The listing builds one solid part. Answer for the finished solid, in the listing's coordinates (mm). A direction names the side the tool comes from. Coordinates: 2 decimals unless noted, no trailing zeros. Write each loop counter-clockwise with the first axis right and the second up, starting at its lowest first coordinate (ties: lowest second). Pieces come first, ordered by that corner, then holes.
from build123d import *
from build123d.topology import SkipClean

# Parameters (mm, degrees)
SKETCH_1_W          = 60
SKETCH_1_H          = 60
EXTRUDE_1_DEPTH     = 5
EXTRUDE_START       = 5
SKETCH_2_R          = 17.67766953
EXTRUDE_3_DEPTH     = 10
SKETCH_6_W          = 30
SKETCH_6_H          = 30
CUT_EXTRUDE_2_DEPTH = 5
CHAMFER_1_SIZE      = 5
SKETCH_7_R          = 6.25
EXTRUDE_4_DEPTH     = 7
CUT_EXTRUDE_START   = 5
CUT_EXTRUDE_3_DEPTH = 5
CUT_EXTRUDE_4_DEPTH = 7
SKETCH_18_R         = 2.5
CUT_EXTRUDE_5_DEPTH = 12
SKETCH_21_R         = 2.5
CUT_EXTRUDE_6_DEPTH = 10
FILLET_1_R          = 1
FILLET_2_R          = 3


with BuildPart() as part:
    # 草图1 → 凸台-拉伸1 (new body)
    with BuildSketch(Plane(origin=(0, 0, 0), x_dir=(1, 0, 0), z_dir=(0, 1, 0))):
        Rectangle(SKETCH_1_W, SKETCH_1_H)
    extrude(amount=EXTRUDE_1_DEPTH)

    # 草图2 → 凸台-拉伸3 (add)
    with BuildSketch(Plane(origin=(0, 0, 0), x_dir=(1, 0, 0), z_dir=(0, 1, 0)).offset(EXTRUDE_START)):
        with Locations(Location((0, 0, 0), (0, 0, 90))):
            Circle(SKETCH_2_R)
    extrude(amount=EXTRUDE_3_DEPTH)

    # 扫描1: sweep along a curve in space
    with BuildLine() as sweep_1_path:
        ThreePointArc((0, 5, -17.67766953), (12.5, 5, -12.5), (17.67766953, 5, 0))
        ThreePointArc((17.67766953, 5, 0), (12.5, 5, 12.5), (0, 5, 17.67766953))
        ThreePointArc((0, 5, 17.67766953), (-12.5, 5, 12.5), (-17.67766953, 5, 0))
        ThreePointArc((-17.67766953, 5, 0), (-12.5, 5, -12.5), (0, 5, -17.67766953))
    # 草图4 → 扫描1 (sweep)
    with BuildSketch(Plane.XY):
        Polygon((17.67766953, 15), (17.67766953, 5), (27.67766953, 5), align=None)
    sweep(path=sweep_1_path.line)

    # 草图6 → 切除-拉伸2 (cut)
    with BuildSketch(Plane(origin=(0, 0, 0), x_dir=(1, 0, 0), z_dir=(0, 1, 0))):
        Rectangle(SKETCH_6_W, SKETCH_6_H)
    extrude(amount=CUT_EXTRUDE_2_DEPTH, mode=Mode.SUBTRACT)

    # 倒角1
    chamfer_1_edges = [part.edges().sort_by_distance(p)[0] for p in [
        (0, 5, -15),
        (-15, 5, 0),
        (0, 5, 15),
        (15, 5, 0),
    ]]
    chamfer(chamfer_1_edges, length=CHAMFER_1_SIZE - 0.0001)  # a hair under: the kernel refuses the full size

    # 草图7 → 凸台-拉伸4 (add)
    with BuildSketch(Plane(origin=(0, 0, 0), x_dir=(1, 0, 0), z_dir=(0, 1, 0))):
        with Locations(Location((-23.75, 23.75, 0), (0, 0, 270))):
            Circle(SKETCH_7_R)
        with Locations(Location((23.75, 23.75, 0), (0, 0, 270))):
            Circle(SKETCH_7_R)
        with Locations(Location((-23.75, -23.75, 0), (0, 0, 270))):
            Circle(SKETCH_7_R)
        with Locations(Location((23.75, -23.75, 0), (0, 0, 270))):
            Circle(SKETCH_7_R)
    extrude(amount=-EXTRUDE_4_DEPTH)

    # 草图8 → 切除-拉伸3 (cut)
    with BuildSketch(Plane(origin=(0, 0, 0), x_dir=(1, 0, 0), z_dir=(0, 1, 0)).offset(CUT_EXTRUDE_START)):
        with BuildLine():
            Line((23.75, 30), (30, 30))
            Line((30, 30), (30, 23.75))
            ThreePointArc((30, 23.75), (28.169417382, 28.169417382), (23.75, 30))
        make_face()
        with BuildLine():
            Line((-30, 30), (-23.75, 30))
            ThreePointArc((-23.75, 30), (-28.169417382, 28.169417382), (-30, 23.75))
            Line((-30, 23.75), (-30, 30))
        make_face()
        with BuildLine():
            Line((-23.75, -30), (-30, -30))
            Line((-30, -30), (-30, -23.75))
            ThreePointArc((-30, -23.75), (-28.169417382, -28.169417382), (-23.75, -30))
        make_face()
        with BuildLine():
            Line((30, -23.75), (30, -30))
            Line((30, -30), (23.75, -30))
            ThreePointArc((23.75, -30), (28.169417382, -28.169417382), (30, -23.75))
        make_face()
    extrude(amount=-CUT_EXTRUDE_3_DEPTH, mode=Mode.SUBTRACT)

    # 草图9 → 旋转1 (revolve)
    with BuildSketch(Plane(origin=(0, 0, 23.75), x_dir=(-1, 0, 0), z_dir=(0, 0, -1)), mode=Mode.PRIVATE) as revolve_1_sk:
        Polygon((17.5, -7), (17.5, 0), (12.5, 0), align=None)
    revolve(revolve_1_sk.sketch.rotate(Axis((-23.75, 5, 23.75), (0, -1, 0)), 90), axis=Axis((-23.75, 5, 23.75), (0, -1, 0)))

    # 草图13 → 旋转2 (revolve)
    with BuildSketch(Plane(origin=(0, 0, 23.75), x_dir=(-1, 0, 0), z_dir=(0, 0, -1)), mode=Mode.PRIVATE) as revolve_2_sk:
        Polygon((-17.5, 0), (-17.5, -7), (-12.5, 0), align=None)
    revolve(revolve_2_sk.sketch.rotate(Axis((23.75, 5, 23.75), (0, -1, 0)), 270), axis=Axis((23.75, 5, 23.75), (0, -1, 0)))

    # 草图14 → 旋转3 (revolve)
    with BuildSketch(Plane(origin=(0, 0, -23.75), x_dir=(-1, 0, 0), z_dir=(0, 0, -1)), mode=Mode.PRIVATE) as revolve_3_sk:
        Polygon((-17.5, -7), (-12.5, 0), (-17.5, 0), align=None)
    revolve(revolve_3_sk.sketch.rotate(Axis((23.75, 5, -23.75), (0, -1, 0)), 270), axis=Axis((23.75, 5, -23.75), (0, -1, 0)))

    # 草图16 → 旋转4 (revolve)
    with BuildSketch(Plane(origin=(0, 0, -23.75), x_dir=(-1, 0, 0), z_dir=(0, 0, -1)), mode=Mode.PRIVATE) as revolve_4_sk:
        Polygon((17.5, 0), (17.5, -7), (12.5, 0), align=None)
    revolve(revolve_4_sk.sketch.rotate(Axis((-23.75, 5, -23.75), (0, -1, 0)), 90), axis=Axis((-23.75, 5, -23.75), (0, -1, 0)))

    # 草图17 → 切除-拉伸4 (cut)
    with SkipClean():  # the faces are left unmerged after this step: merging them gives an invalid solid
        with BuildSketch(Plane(origin=(0, 0, 0), x_dir=(1, 0, 0), z_dir=(0, 1, 0))):
            with BuildLine():
                Line((-30, -23.75), (-30, -14.395856533))
                ThreePointArc((-30, -14.395856533), (-31.704951288, -31.704951288), (-14.395856533, -30))
                Line((-14.395856533, -30), (-23.75, -30))
                ThreePointArc((-23.75, -30), (-28.169417382, -28.169417382), (-30, -23.75))
            make_face()
            with BuildLine():
                Line((30, -14.395856533), (30, -23.75))
                ThreePointArc((30, -23.75), (28.169417382, -28.169417382), (23.75, -30))
                Line((23.75, -30), (14.395856533, -30))
                ThreePointArc((14.395856533, -30), (31.704951288, -31.704951288), (30, -14.395856533))
            make_face()
            with BuildLine():
                Line((30, 23.75), (30, 14.395856533))
                ThreePointArc((30, 14.395856533), (31.704951288, 31.704951288), (14.395856533, 30))
                Line((14.395856533, 30), (23.75, 30))
                ThreePointArc((23.75, 30), (28.169417382, 28.169417382), (30, 23.75))
            make_face()
            with BuildLine():
                Line((-23.75, 30), (-14.395856533, 30))
                ThreePointArc((-14.395856533, 30), (-31.704951288, 31.704951288), (-30, 14.395856533))
                Line((-30, 14.395856533), (-30, 23.75))
                ThreePointArc((-30, 23.75), (-28.169417382, 28.169417382), (-23.75, 30))
            make_face()
        extrude(amount=-CUT_EXTRUDE_4_DEPTH, mode=Mode.SUBTRACT)

    # 草图18 → 切除-拉伸5 (cut)
    with SkipClean():  # the faces are left unmerged after this step: merging them gives an invalid solid
        with BuildSketch(Plane(origin=(0, 0, 0), x_dir=(1, 0, 0), z_dir=(0, 1, 0)).offset(CUT_EXTRUDE_START)):
            with Locations(Location((-23.75, 23.75, 0), (0, 0, 270))):
                Circle(SKETCH_18_R)
            with Locations(Location((23.75, 23.75, 0), (0, 0, 270))):
                Circle(SKETCH_18_R)
            with Locations(Location((-23.75, -23.75, 0), (0, 0, 270))):
                Circle(SKETCH_18_R)
            with Locations(Location((23.75, -23.75, 0), (0, 0, 270))):
                Circle(SKETCH_18_R)
        extrude(amount=-CUT_EXTRUDE_5_DEPTH, mode=Mode.SUBTRACT)

    # 草图21 → 切除-拉伸6 (cut)
    with SkipClean():  # the faces are left unmerged after this step: merging them gives an invalid solid
        with BuildSketch(Plane(origin=(0, 0, 0), x_dir=(1, 0, 0), z_dir=(0, 1, 0)).offset(CUT_EXTRUDE_START)):
            with Locations(Location((-6, 6, 0), (0, 0, 90))):
                Circle(SKETCH_21_R)
            with Locations(Location((6, 6, 0), (0, 0, 90))):
                Circle(SKETCH_21_R)
            with Locations(Location((6, -6, 0), (0, 0, 90))):
                Circle(SKETCH_21_R)
            with Locations(Location((-6, -6, 0), (0, 0, 90))):
                Circle(SKETCH_21_R)
        extrude(amount=CUT_EXTRUDE_6_DEPTH, mode=Mode.SUBTRACT)

    # 圆角1
    fillet_1_edges = [part.edges().sort_by_distance(p)[0] for p in [
        (0, 5, 30),
        (-30, 5, 0),
        (0, 5, -30),
        (30, 5, 0),
        (28.169417382, 5, 28.169417382),
        (-28.169417382, 5, 28.169417382),
        (-28.169417382, 5, -28.169417382),
        (28.169417382, 5, -28.169417382),
    ]]
    fillet(fillet_1_edges, radius=FILLET_1_R)

    # 圆角2
    fillet_2_edges = [part.edges().sort_by_distance(p)[0] for p in [
        (0, 15, -17.67766953),
        (-12.5, 15, 12.5),
    ]]
    fillet(fillet_2_edges, radius=FILLET_2_R)


solid = part.part
1. For a pull along X with two mould halves and no side action, classify faces 3 (the flat face through (-11, 5, 26)), 4 (the flat face through (30, 1, 0)), 5 (the cylindrical face through (5.249, 9.93, -8.385)) as pulls with the +X half, pulls with the -X half, needs draft (parallel to the pull), parting line crosses it, or undercut.
Results found:
face 3: needs draft
face 4: pulls with the +X half
face 5: undercut
2. A tool of negligible diameter and unlimited length cuts with its end or side. For faces 1 (the cylindrical face through (25.44, -0.92, -25.59)), 2 (the flat face through (0, 3, -12)), from which of +Z, -Z, +X, -X, +Y, -Y can it reach the whole face along a straight path? Write none if from no direction.
Results found:
face 1: +Y, -Y
face 2: -Y
3. Flat-ended cylindrical pins translate along their axes: P1, Ø3, axis at x = 11, z = 16.5, coming from the +Y side; P2, Ø4, axis at y = 11.5, z = -2, coming from the +X side; P3, Ø18, axis at x = -4.5, z = 13.5, coming from the -Y side; P4, Ø3, axis at x = 6, z = 6, coming from the -Y side. Find the tip coordinate at first contact, or state that the pin passes through.
Results found:
P1: stops at y = 14.33
P2: stops at x = 23.1
P3: stops at y = 0
P4: passes through
4. Find the intervals of material crossed by L1, parallel to X at y = 14, z = -6.5; L2, parallel to X at y = -5, z = -26; L3, parallel to X at y = -3.25, z = -23.75, in increasing order.
Results found:
L1: x = -17.51 to -8.45, -3.55 to 3.55, 8.45 to 17.51
L2: x = -29.58 to -24.84, -22.66 to -16.41, 16.41 to 22.66, 24.84 to 29.58
L3: x = -30 to -26.25, -21.25 to -14.82, 14.82 to 21.25, 26.25 to 30
5. Section B-B on y = 8.75 is taken. Give the vertices of the cut face in (x, z), then the cut area to 3 significant figures.
Results found:
outline: circle Ø47.86 at (0, 0); hole circle Ø5 at (-6, -6); hole circle Ø5 at (-6, 6); hole circle Ø5 at (6, -6); hole circle Ø5 at (6, 6)
area: 1,720 mm2
6. Section C-C on x = 6 is taken. State how many separate pieces and enclosed holes the cut face has, then the cut area to 3 significant figures.
Results found:
separate pieces: 3
enclosed holes: 0
area: 511 mm2
